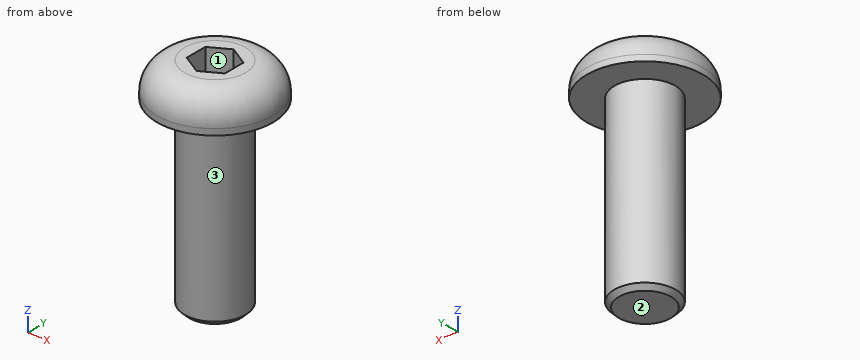
from build123d import *

# Parameters (mm, degrees)
SKETCH1_R           = 3.8
BOSS_EXTRUDE1_DEPTH = 2.2
SKETCH2_R           = 2
BOSS_EXTRUDE2_DEPTH = 12
CHAMFER1_SIZE       = 0.3
CUT_EXTRUDE1_DEPTH  = 2
FILLET1_R           = 1.8


with BuildPart() as part:
    # Sketch1 → Boss-Extrude1 (new body)
    with BuildSketch(Plane.XY):
        Circle(SKETCH1_R)
    extrude(amount=BOSS_EXTRUDE1_DEPTH)

    # Sketch2 → Boss-Extrude2 (add)
    with BuildSketch(Plane(origin=(0, 0, 0), x_dir=(-1, 0, 0), z_dir=(0, 0, -1))):
        Circle(SKETCH2_R)
    extrude(amount=BOSS_EXTRUDE2_DEPTH)

    # Chamfer1
    chamfer1_edges = [part.edges().sort_by_distance(p)[0] for p in [
        (2, 0, -12),
    ]]
    chamfer(chamfer1_edges, length=CHAMFER1_SIZE)

    # Sketch3 → Cut-Extrude1 (cut)
    with BuildSketch(Plane.XY.offset(2.2)):
        Polygon((0, 1.443375673), (-1.25, 0.721687836), (-1.25, -0.721687836), (0, -1.443375673), (1.25, -0.721687836), (1.25, 0.721687836), align=None)
    extrude(amount=-CUT_EXTRUDE1_DEPTH, mode=Mode.SUBTRACT)

    # Fillet1
    fillet1_edges = [part.edges().sort_by_distance(p)[0] for p in [
        (-3.8, 0, 2.2),
    ]]
    fillet(fillet1_edges, radius=FILLET1_R)


solid = part.part
Here's how the part is built. I have some questions about the finished solid (model axes, mm). Face numbers are marked on the shaded views. Coordinates: 2 decimals unless noted, no trailing zeros. Order: outer loops, then holes, each group sorted by start corner. A loop starts at its lowest first (then second) coordinate and runs counter-clockwise, first axis right, second up. Notation, with made-up numbers: M -10.5,19.5 L 37.5,19.5 A21 cw 37.5,44.5 Z; hole C 38,-12 d7. An arc over 180 degrees is marked long. Answer as CSV lines item,"result". Start each with the question number.
1. I want a section at B-B, the plane z = -9.75. Write out the boundary of the cut face in (x, y).
2. I want a section at A-A, the plane y = 0. Write out the boundary of the cut face in (x, z), and give its area (3 significant figures).
3. I need wall thicknesses on line 1 (Z direction, x = 2, y = -2); line 2 (Y direction, x = 0.75, z = 0.75); line 3 (Z direction, x = 0, y = 0.5). Which ranges of each line are inside material? Lowest first, please. Write a range as [from, to].
4. We'd pull the mould along X, two halves only. Please class the marked faces 1, 2 and 3: released by +X, released by -X, zero draft, split by the parting line, or undercut.
5. For pin 1 (4 mm diameter, centred on x = -3, z = -5.5, fed in from -Y); pin 2 (1 mm diameter, centred on x = 2, z = -6, fed in from -Y); pin 3 (0.7 mm diameter, centred on y = 0, z = 1, fed in from -X); pin 4 (1.5 mm diameter, centred on x = -3, z = -8.5, fed in from +Y), each with a flat end and sliding along its axis, tell me the tip position at first contact or that it passes through.
Recorded:
1,outline,"C 0,0 d4"
2,outline,"M -3.8,0 L -2,0 L -2,-11.7 L -1.7,-12 L 1.7,-12 L 2,-11.7 L 2,0 L 3.8,0 L 3.8,0.4 A1.8 ccw 2,2.2 L 1.25,2.2 L 1.25,0.2 L -1.25,0.2 L -1.25,2.2 L -2,2.2 A1.8 ccw -3.8,0.4 Z"
2,area,"58.2 mm2"
3,line 1,"z = [0, 2]"
3,line 2,"y = [-3.69, -1.01], [1.01, 3.69]"
3,line 3,"z = [-12, 0.2]"
4,face 1,"undercut"
4,face 2,"zero draft"
4,face 3,"split by the parting line"
5,pin 1,"stops at y = -1.73"
5,pin 2,"stops at y = -1.32"
5,pin 3,"stops at x = -3.78"
5,pin 4,"passes through"
